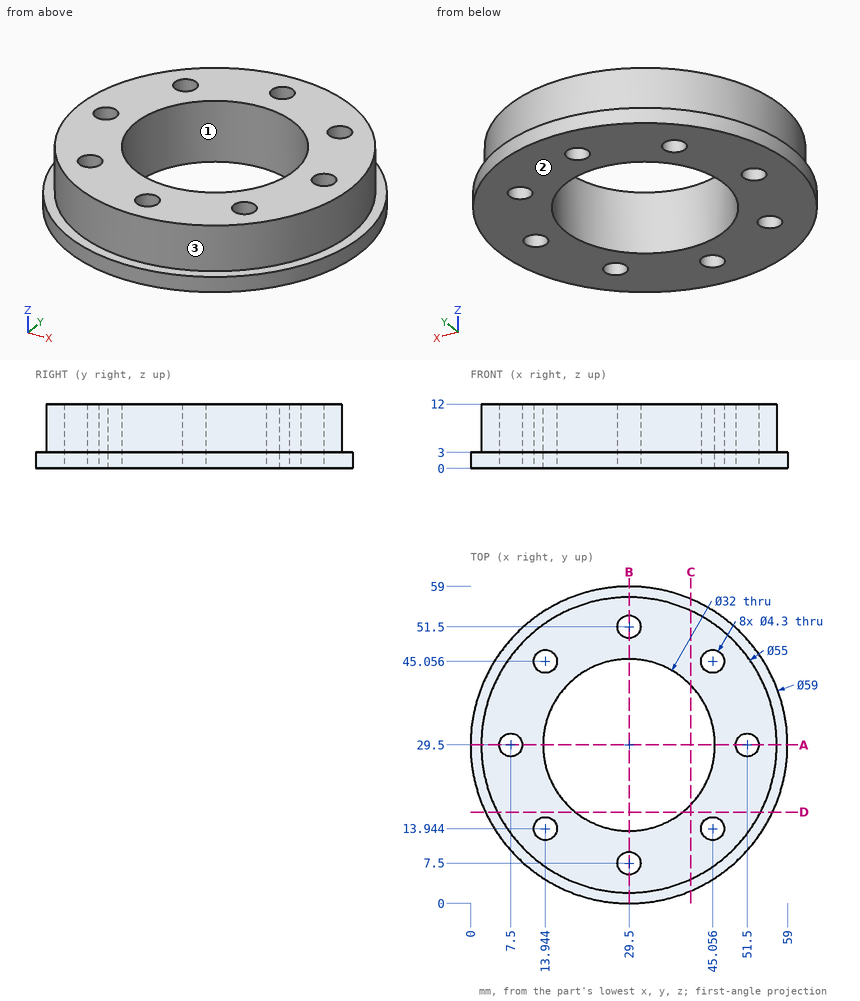
Design review of the part shown in the three views and the two pictorial views. Dimensions are in mm from the part's minimum x, y and z. Coordinates: 2 decimals unless noted, no trailing zeros. Loops run counter-clockwise (first coordinate to the right, second up) from the corner with the lowest first, then second, coordinate; pieces in that order, holes last. Notation, with made-up numbers: (-16.5, 39) - (37.5, 39) arc R28 cw to (37.5, 59) - close; hole circle Ø2 at (-18, 35.5). An arc over 180 degrees is marked (long way). Use a Markdown table: item, result. Add a question column.
Item 1: We need section C-C (x = 41). Give the boundary of the cut face in (y, z).
Item 2: Insertion check: pin 1 Ø4 at (x, y) = (20, 20.5) entering from -Z; pin 2 Ø1.5 at (y, z) = (52.5, 4.5) entering from +X; pin 3 Ø3 at (x, y) = (48, 53) entering from +Z; pin 4 Ø6 at (x, z) = (45, 5.5) entering from -Y. Each pin has a flat end and moves straight along its axis. Give the tip position at first contact, or say it passes through.
Item 3: We need section A-A (y = 29.5). Give the boundary of the cut face in (x, z).
Item 4: We need section D-D (y = 17). Give the boundary of the cut face in (x, z) (1 decimal).
Item 5: Mouldability with a two-part tool opening along X and no side actions: class the marked faces 1, 2 and 3 as pulls with the +X half, pulls with the -X half, needs draft (parallel to the pull), parting line crosses it, or undercut.
Item 6: For line 1 (X direction, y = 29.5, z = 3.5); line 2 (X direction, y = 15.5, z = 6.5) (1 decimal); line 3 (X direction, y = 21.5, z = 10), list the stretches that pass through material, from the lowest coordinate up.
Results list:
| question | item | result |
|---|---|---|
| 1 | outline | (2.33, 0) - (18.38, 0) - (18.38, 12) - (4.52, 12) - (4.52, 3) - (2.33, 3) - close; (40.62, 0) - (56.67, 0) - (56.67, 3) - (54.48, 3) - (54.48, 12) - (40.62, 12) - close |
| 2 | pin 1 | passes through |
| 2 | pin 2 | stops at x = 45.66 |
| 2 | pin 3 | stops at z = 3 |
| 2 | pin 4 | stops at y = 3.45 |
| 3 | outline | (0, 0) - (5.35, 0) - (5.35, 12) - (2, 12) - (2, 3) - (0, 3) - close; (9.65, 0) - (13.5, 0) - (13.5, 12) - (9.65, 12) - close; (45.5, 0) - (49.35, 0) - (49.35, 12) - (45.5, 12) - close; (53.65, 0) - (59, 0) - (59, 3) - (57, 3) - (57, 12) - (53.65, 12) - close |
| 4 | outline | (2.8, 0) - (19.5, 0) - (19.5, 12) - (5, 12) - (5, 3) - (2.8, 3) - close; (39.5, 0) - (56.2, 0) - (56.2, 3) - (54, 3) - (54, 12) - (39.5, 12) - close |
| 5 | face 1 | undercut |
| 5 | face 2 | needs draft |
| 5 | face 3 | parting line crosses it |
| 6 | line 1 | x = 2 to 5.35, 9.65 to 13.5, 45.5 to 49.35, 53.65 to 57 |
| 6 | line 2 | x = 5.8 to 12.5, 15.4 to 21.8, 37.2 to 43.6, 46.5 to 53.2 |
| 6 | line 3 | x = 3.19 to 15.64, 43.36 to 55.81 |
